The listing builds one solid part. Answer for the finished solid, in the listing's coordinates (mm). Round coordinates to 2 decimals unless told otherwise and drop trailing zeros. Order: outer loops, then holes, each group sorted by start corner. A loop starts at its lowest first (then second) coordinate and runs counter-clockwise, first axis right, second up. Notation, with made-up numbers: M -35,34 L -15,34 A14 ccw -15,38 Z; hole C -17.75,51 d11. An arc over 180 degrees is marked long. Put each result on its own line as item: value. Start each with the question number.
1. The part is cut by section A-A (z = 439). Give the vertices of the cut face in (x, y) (3 decimals), then the cut area to 3 significant figures.
2. Consider line 1 (Y direction, x = 0, z = 647.75); line 2 (X direction, y = 0, z = 240.5); line 3 (Y direction, x = 0, z = 186). Determine where each line is inside the solid, lowest interval first.
3. Each of these flat-tipped pins is pushed along its axis until it touches: pin 1 Ø4 at (y, z) = (2, 262) entering from +X; pin 2 Ø1.5 at (x, z) = (-3, 481) entering from +Y; pin 3 Ø4.5 at (x, y) = (0, 0) entering from -Z. Where does it stop, or does it pass through?
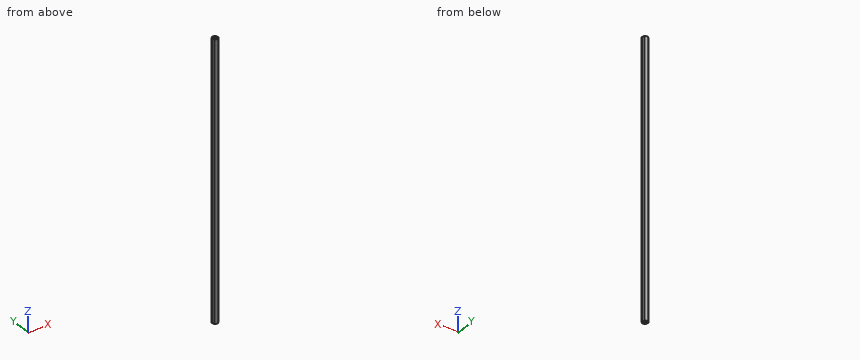
from build123d import *

# Parameters (mm, degrees)
BOSS_EXTRUDE1_DEPTH         = 658.9014
SKETCH2_R                   = 2.0193
CUT_EXTRUDE1_DEPTH          = 659.969574666
F_1_4_20_TAPPED_HOLE1_D     = 5.1054
F_1_4_20_TAPPED_HOLE1_DEPTH = 19.05
F_1_4_20_TAPPED_HOLE1_TIP   = 1.533816902
F_1_4_20_TAPPED_HOLE2_D     = 5.1054
F_1_4_20_TAPPED_HOLE2_DEPTH = 19.05
F_1_4_20_TAPPED_HOLE2_TIP   = 1.533816902


with BuildPart() as part:
    # Sketch1 → Boss-Extrude1 (new body)
    with BuildSketch(Plane.XY):
        with BuildLine():
            Line((-6.654540832, 1.131188008), (-5.845671476, -3.375))
            ThreePointArc((-5.845671476, -3.375), (-5.15742276, -4.354709), (-4.306907968, -5.197407407))
            Line((-4.306907968, -5.197407407), (0, -6.75))
            ThreePointArc((0, -6.75), (1.19257724, -6.643813628), (2.347632865, -6.328595415))
            Line((2.347632865, -6.328595415), (5.845671476, -3.375))
            ThreePointArc((5.845671476, -3.375), (6.35, -2.289104628), (6.654540832, -1.131188008))
            Line((6.654540832, -1.131188008), (5.845671476, 3.375))
            ThreePointArc((5.845671476, 3.375), (5.15742276, 4.354709), (4.306907968, 5.197407407))
            Line((4.306907968, 5.197407407), (0, 6.75))
            ThreePointArc((0, 6.75), (-1.19257724, 6.643813628), (-2.347632865, 6.328595415))
            Line((-2.347632865, 6.328595415), (-5.845671476, 3.375))
            ThreePointArc((-5.845671476, 3.375), (-6.35, 2.289104628), (-6.654540832, 1.131188008))
        make_face()
    extrude(amount=BOSS_EXTRUDE1_DEPTH)

    # Sketch2 → Cut-Extrude1 (cut, through all)
    with BuildSketch(Plane.XY.offset(658.9014)):
        Circle(SKETCH2_R)
    extrude(amount=-CUT_EXTRUDE1_DEPTH, mode=Mode.SUBTRACT)

    # 1/4-20 Tapped Hole1
    with Locations(Plane.XY.offset(658.9014)):
        with Locations((0, 0)):
            Hole(F_1_4_20_TAPPED_HOLE1_D / 2, depth=F_1_4_20_TAPPED_HOLE1_DEPTH)
            with Locations((0, 0, -(F_1_4_20_TAPPED_HOLE1_DEPTH + F_1_4_20_TAPPED_HOLE1_TIP / 2))):  # 118° drill point
                Cone(0, F_1_4_20_TAPPED_HOLE1_D / 2, F_1_4_20_TAPPED_HOLE1_TIP, mode=Mode.SUBTRACT)

    # 1/4-20 Tapped Hole2
    with Locations(Plane(origin=(0, 0, 0), x_dir=(-1, 0, 0), z_dir=(0, 0, -1))):
        with Locations((0, 0)):
            Hole(F_1_4_20_TAPPED_HOLE2_D / 2, depth=F_1_4_20_TAPPED_HOLE2_DEPTH)
            with Locations((0, 0, -(F_1_4_20_TAPPED_HOLE2_DEPTH + F_1_4_20_TAPPED_HOLE2_TIP / 2))):  # 118° drill point
                Cone(0, F_1_4_20_TAPPED_HOLE2_D / 2, F_1_4_20_TAPPED_HOLE2_TIP, mode=Mode.SUBTRACT)


solid = part.part
Resolved:
1. outline: M -6.655,1.131 L -5.846,-3.375 A6.75 ccw -4.307,-5.197 L 0,-6.75 A6.75 ccw 2.348,-6.329 L 5.846,-3.375 A6.75 ccw 6.655,-1.131 L 5.846,3.375 A6.75 ccw 4.307,5.197 L 0,6.75 A6.75 ccw -2.348,6.329 L -5.846,3.375 A6.75 ccw Z; hole C 0,0 d4.039
1. area: 123 mm2
2. line 1: -6.75 to -2.55, 2.55 to 6.75
2. line 2: -6.45 to -2.02, 2.02 to 6.45
2. line 3: -6.75 to -2.02, 2.02 to 6.75
3. pin 1: x = 6.45
3. pin 2: y = 6.36
3. pin 3: z = 19.23
